Read the model definition and answer for the solid it produces. Units are mm, in the model's axes. Coordinates: 2 decimals unless noted, no trailing zeros. Loops run counter-clockwise (first coordinate to the right, second up) from the corner with the lowest first, then second, coordinate; pieces in that order, holes last. Notation, with made-up numbers: (69, 55.5) - (88, 55.5) arc R27 ccw to (88, 91.5) - close; hole circle Ø4 at (-1.75, 80). An arc over 180 degrees is marked (long way). Use one line per item in the form item = value.
from build123d import *

# Parameters (mm, degrees)
EXTRUDE_1_DEPTH      = 30
EXTRUDE_1_DEPTH_BACK = 30
SKETCH_1_W           = 38
SKETCH_1_H           = 3
SKETCH_2_R           = 5
SKETCH_2_W           = 32
SKETCH_2_H           = 8
CUT_EXTRUDE_1_DEPTH  = 51.089919145


with BuildPart() as part:
    # Эскиз1 → Бобышка-Вытянуть1 (new, two sides: drawn at the far end of the back side and taken through both)
    with BuildSketch(Plane(origin=(0, 0, 0), x_dir=(0, 0, -1), z_dir=(1, 0, 0)).offset(-EXTRUDE_1_DEPTH_BACK)):
        with Locations((-21, 9.245966692)):
            Rectangle(SKETCH_1_W, SKETCH_1_H)
    extrude(amount=EXTRUDE_1_DEPTH + EXTRUDE_1_DEPTH_BACK)

    # Эскиз2 → Вырез-Вытянуть1 (cut, through all)
    with BuildSketch(Plane(origin=(0, 10.745966692, 0), x_dir=(1, 0, 0), z_dir=(0, 1, 0))):
        with Locations(Location((-20, -21, 0), (0, 0, 270))):
            Circle(SKETCH_2_R)
        with Locations(Location((20, -21, 0), (0, 0, 270))):
            Circle(SKETCH_2_R)
        with Locations((14, -6)):
            Rectangle(SKETCH_2_W, SKETCH_2_H)
    extrude(amount=-CUT_EXTRUDE_1_DEPTH, mode=Mode.SUBTRACT)


solid = part.part
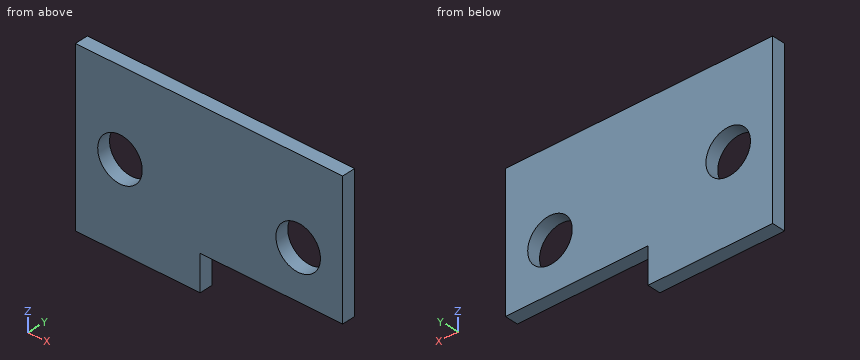
Item 1: Find the intervals of material crossed by L1, parallel to X at y = 8.6, z = 21; L2, parallel to X at y = 9.05, z = 25; L3, parallel to Z at x = -23.5, y = 9.4, in increasing order.
Results below:
L1 = -30 to -25, -15 to 15, 25 to 30
L2 = -30 to -23, -17 to 17, 23 to 30
L3 = 2 to 17.43, 24.57 to 40
Item 2: Each of these flat-tipped pins is pushed along its axis until it touches: P1, Ø1.5, axis at x = 15, y = 9, coming from the -Z side; P2, Ø11.5, axis at x = -20, z = 21, coming from the +Y side; P3, Ø1.5, axis at y = 9.5, z = 6, coming from the +X side. Where does it stop, or does it pass through?
Results below:
P1 = 10
P2 = 10.75
P3 = -2
Item 3: The part is cut by section D-D on x = 20. Give the vertices of the cut face in (y, z).
Results below:
outline = (7.75, 10) - (10.75, 10) - (10.75, 16) - (7.75, 16) - close; (7.75, 26) - (10.75, 26) - (10.75, 40) - (7.75, 40) - close
Item 4: The part is cut by section C-C on y = 8.4. Give the vertices of the cut face in (x, z).
Results below:
outline = (-30, 2) - (-2, 2) - (-2, 10) - (30, 10) - (30, 40) - (-30, 40) - close; hole circle Ø10 at (-20, 21); hole circle Ø10 at (20, 21)
Item 5: The part is cut by section B-B on z = 21. Give the vertices of the cut face in (x, y).
Results below:
outline = (-30, 7.75) - (-25, 7.75) - (-25, 10.75) - (-30, 10.75) - close; (-15, 7.75) - (15, 7.75) - (15, 10.75) - (-15, 10.75) - close; (25, 7.75) - (30, 7.75) - (30, 10.75) - (25, 10.75) - close
Item 6: The part is cut by section A-A on x = -20. Give the vertices of the cut face in (y, z).
Results below:
outline = (7.75, 2) - (10.75, 2) - (10.75, 16) - (7.75, 16) - close; (7.75, 26) - (10.75, 26) - (10.75, 40) - (7.75, 40) - close
